Autodesk Fusion 360 part; units mm, degrees
sketch "Sketch1" plane through (0, 0, 0) normal (0, 0, 1) x (1, 0, 0)
  circle A0 centre (0, 0) radius 8
  circle A1 centre (0, 0) radius 4
  dimension "d1" = 16
  dimension "d2" = 8
extrude "Extrude1" add sketch "Sketch1" along normal blind 5
sketch "Sketch2" plane through (0, 0, 5) normal (0, 0, 1) x (-1, 0, 0)
  circle A0 centre (0, 0) radius 4
  circle A1 centre (0, 0) radius 8
  circle A2 centre (0, 0) radius 7
  circle A3 centre (0, 0) radius 5
  dimension "d5" = -1
  dimension "d6" = 1
extrude "Extrude2" cut sketch "Sketch2" against normal blind 0.5 contours A2
sketch "Sketch3" plane through (0, 0, 0) normal (0, 0, -1) x (1, 0, 0)
  circle A0 centre (0, 0) radius 4
  circle A1 centre (0, 0) radius 8
  circle A2 centre (0, 0) radius 5
  circle A3 centre (0, 0) radius 7
extrude "Extrude3" cut sketch "Sketch3" against normal blind 0.5 contours A3
Design review of the part built by this model. Coordinates are the model's own, in mm. A direction names the side the tool comes from. Round coordinates to 2 decimals unless told otherwise and drop trailing zeros. Loops run counter-clockwise (first coordinate to the right, second up) from the corner with the lowest first, then second, coordinate; pieces in that order, holes last. Notation, with made-up numbers: M 67.25,12 L 113.25,12 A19 cw 113.25,47 Z; hole C 89,81.5 d5. An arc over 180 degrees is marked long. Answer as a JSON object with one key per item and string values.
Item 1: We need section A-A on x = 0. Give the boundary of the cut face in (y, z).
Answer sheet:
{"outline": "M -8,0 L -7,0 L -7,0.5 L -5,0.5 L -5,0 L -4,0 L -4,5 L -5,5 L -5,4.5 L -7,4.5 L -7,5 L -8,5 Z; M 4,0 L 5,0 L 5,0.5 L 7,0.5 L 7,0 L 8,0 L 8,5 L 7,5 L 7,4.5 L 5,4.5 L 5,5 L 4,5 Z"}
Item 2: Clearance check with flat-ended pins moving along their axes: P1, Ø1, axis at y = -0.5, z = 1, coming from the +X side; P2, Ø1, axis at x = 3.5, z = 1.5, coming from the +Y side; P3, Ø1, axis at x = -2.5, y = 5, coming from the +Z side. State where each tip first meets the part, or that it passes through.
Answer sheet:
{"P1": "stops at x = 8", "P2": "stops at y = 7.42", "P3": "stops at z = 4.5"}
Item 3: We need section C-C on z = 1.3. Give the boundary of the cut face in (x, y), and give its area (3 significant figures).
Answer sheet:
{"outline": "C 0,0 d16; hole C 0,0 d8", "area": "151 mm^2"}
Item 4: The part is to be moulded in two halves that separate along X. For faces 1 (the cylindrical face through (-1.73, 7.81, 2.46)), 2 (the flat face through (-2, -5, 0.5)), 3 (the flat face through (4, -6, 5)), say which applies: pulls with the +X half, pulls with the -X half, needs draft (parallel to the pull), parting line crosses it, or undercut.
Answer sheet:
{"face 1": "parting line crosses it", "face 2": "undercut", "face 3": "needs draft"}
Item 5: We need section D-D on y = -5.75. Give the boundary of the cut face in (x, z).
Answer sheet:
{"outline": "M -5.56,0 L -3.99,0 L -3.99,0.5 L 3.99,0.5 L 3.99,0 L 5.56,0 L 5.56,5 L 3.99,5 L 3.99,4.5 L -3.99,4.5 L -3.99,5 L -5.56,5 Z"}
Item 6: Machinability: for faces 4 (the cylindrical face through (6.466, 2.681, 0.246)), 5 (the flat face through (4, -6, 0)), 6 (the flat face through (2, -5, 4.5)), which of the approach directions +Z, -Z, +X, -X, +Y, -Y give a long, thin tool a straight path to every point of the face, cutting with its end or side? Answer none if there is none.
Answer sheet:
{"face 4": "-Z", "face 5": "-Z, +X, -X, +Y, -Y", "face 6": "+Z"}
Item 7: Wall thickness on L1, parallel to Y at x = 0, z = 0.45; L2, parallel to Y at x = 0, z = 2.95; L3, parallel to Y at x = 3.25, z = 1.85: over which ranges is each line inside the solid? List them lowest first. Write a range as from..to.
Answer sheet:
{"L1": "y = -8..-7, -5..-4, 4..5, 7..8", "L2": "y = -8..-4, 4..8", "L3": "y = -7.31..-2.33, 2.33..7.31"}
